Read the model definition and answer for the solid it produces. Units are mm, in the model's axes. A direction names the side the tool comes from. Give positions to 0.01 mm unless a question says otherwise; leave off trailing zeros. Order: outer loops, then holes, each group sorted by start corner. A loop starts at its lowest first (then second) coordinate and runs counter-clockwise, first axis right, second up.
Item 1: The mould has two halves that part along X. Classify faces 4 (the face through (-23.897, -34.973, 6.529)), 5 (the face through (121.398, 23, 13)), 6 (the face through (38.65, 3.02, 2.06)), 7 (the face through (-39.378, 22.614, 2.504)): +X half, -X half, draft (parallel to the pull), parting line (faces both ways), or undercut.
Item 2: Given pin 1 Ø1 at (y, z) = (-45, 17) entering from -X; pin 2 Ø1.5 at (y, z) = (-42, 13) entering from +X; pin 3 Ø1 at (x, z) = (82.5, 16.5) entering from -Y, each flat-ended and moving along its own axis, determine where each tip first touches the part or whether it passes through.
Item 3: Find the intervals of material crossed by line 1 along Y through (x, z) = (54.5, 10.75); line 2 along X through (y, z) = (-28, 18); line 3 along X through (y, z) = (-52.5, 14.5), in increasing order.
Item 4: Which of the six approach directions +Z, -Z, +X, -X, +Y, -Y give full straight-line access (tool end or side, diameter ignored) to faces 1 (the face through (96.987, -33, 13)), 2 (the face through (-35.43, -34.97, 6.61)), 3 (the face through (-38.81, 42.18, 21.93))?
Item 5: A cutting plane is placed at A-A (y = -45.5). Write down the section's boundary in (x, z), plus the area to 3 significant figures.
Item 6: A cutting plane is placed at B-B (x = 14.5). Write down the section's boundary in (y, z), plus the area to 3 significant figures.
from build123d import *

# Parameters (mm, degrees)
F0_W         = 163.3519083261
F0_H         = 45.7251667976
F1_DEPTH     = 25.4
F2_SIZE      = 5.08
F3_W         = 14.5046669376
F3_H         = 15.24
F4_DEPTH     = 70.9391236305
F5_W         = 19.3313653898
F5_H         = 15.24
F6_DEPTH     = 72.0867142081
F7_T1_DEPTH  = 39.9046669376
F7_T6_DEPTH  = 96.3391236305
F7_T12_DEPTH = 96.3391236305
F7_T18_DEPTH = 96.3391236305
F7_T24_DEPTH = 83.6391236305
F7_T29_DEPTH = 83.6391236305
F7_T34_DEPTH = 83.6391236305
F7_T39_DEPTH = 83.6391236305
F7_T44_DEPTH = 96.3391236305
F7_T50_DEPTH = 96.3391236305
F7_T56_DEPTH = 96.3391236305
F8_T1_DEPTH  = 6.4524666085
F8_T3_DEPTH  = 6.4524666085
F8_T5_DEPTH  = 85.150863787
F8_T7_DEPTH  = 45.4596645476
F8_T9_DEPTH  = 41.3682991577
F8_T14_DEPTH = 98.2150133659
F8_T19_DEPTH = 98.2150133659
F8_T24_DEPTH = 98.2150133659
F8_T29_DEPTH = 98.2150133659


# Not quite as in the source:
# - a fillet or chamfer that OpenCascade refuses, or shapes differently, is made with other operations: its cross-section is extruded or revolved along the edge and cut away or added


with BuildPart() as f1:
    # F0 (on Top) → F1 (new body)
    with BuildSketch(Plane.XY):
        with Locations((39.7221744061, 22.8625833988)):
            Rectangle(F0_W, F0_H)
    extrude(amount=F1_DEPTH)

    # F2
    f2_edges = [f1.edges().sort_by_distance(p)[0] for p in [
        (121.398129, 22.862583, 25.4),
        (121.398129, 22.862583, 0),
        (39.722174, 0, 0),
        (121.398129, 0, 12.7),
        (121.398129, 45.725167, 12.7),
        (39.722174, 45.725167, 0),
        (39.722174, 45.725167, 25.4),
        (-41.95378, 22.862583, 25.4),
        (-41.95378, 0, 12.7),
        (-41.95378, 22.862583, 0),
        (-41.95378, 45.725167, 12.7),
        (39.722174, 0, 25.4),
    ]]
    chamfer(f2_edges, length=F2_SIZE)

    # F3 (on face) → F4 (join)
    with BuildSketch(Plane.XZ):
        with Locations((-29.6214462882, 12.7)):
            Rectangle(F3_W, F3_H)
    extrude(amount=F4_DEPTH)

    # F5 (on face) → F6 (join)
    with BuildSketch(Plane.XZ):
        with Locations((106.6524458742, 12.7)):
            Rectangle(F5_W, F5_H)
    extrude(amount=F6_DEPTH)

    # F7: fillet of radius 5.08 on 5 edges, made by hand

    # F7_s2 → F7_t1 (cut)
    with BuildSketch(Plane.YZ.offset(-49.573779757)):
        with BuildLine():
            ThreePointArc((-65.8591236305, 20.32), (-69.451226079, 18.8321024484), (-70.9391236305, 15.24))
            Line((-70.9391236305, 15.24), (-70.9391236305, 20.32))
            Line((-70.9391236305, 20.32), (-65.8591236305, 20.32))
        make_face()
    extrude(amount=F7_T1_DEPTH, mode=Mode.SUBTRACT)


with BuildPart() as f7_tool4:
    # F7_s5 → F7_t6 (new body)
    with BuildSketch(Plane.XZ.offset(-12.7)):
        with BuildLine():
            ThreePointArc((-36.873779757, 15.24), (-35.3858822055, 18.8321024484), (-31.793779757, 20.32))
            Line((-31.793779757, 20.32), (-36.873779757, 20.32))
            Line((-36.873779757, 20.32), (-36.873779757, 15.24))
        make_face()
    extrude(amount=F7_T6_DEPTH)

    split(bisect_by=Plane(origin=(-18.4368898785, -18.4368898785, 0), x_dir=(0, 0, 1), z_dir=(0.7071067812, 0.7071067812, 0)), keep=Keep.TOP)

    split(bisect_by=Plane(origin=(0, -10.16, 10.16), x_dir=(1, 0, 0), z_dir=(0, -0.7071067812, 0.7071067812)), keep=Keep.TOP)


with BuildPart() as f1_1:
    add(f1.part)

    # F7_t3: cut F7_tool4
    add(f7_tool4.part, mode=Mode.SUBTRACT)


with BuildPart() as f7_tool10:
    # F7_s11 → F7_t12 (new body)
    with BuildSketch(Plane.XZ.offset(-12.7)):
        with BuildLine():
            ThreePointArc((-36.873779757, 15.24), (-35.3858822055, 18.8321024484), (-31.793779757, 20.32))
            Line((-31.793779757, 20.32), (-36.873779757, 20.32))
            Line((-36.873779757, 20.32), (-36.873779757, 15.24))
        make_face()
    extrude(amount=F7_T12_DEPTH)

    split(bisect_by=Plane(origin=(-18.4368898785, -18.4368898785, 0), x_dir=(0, 0, 1), z_dir=(-0.7071067812, -0.7071067812, 0)), keep=Keep.TOP)

    split(bisect_by=Plane(origin=(0, -10.16, 10.16), x_dir=(1, 0, 0), z_dir=(0, 0.7071067812, -0.7071067812)), keep=Keep.TOP)


with BuildPart() as f1_2:
    add(f1_1.part)

    # F7_t9: cut F7_tool10
    add(f7_tool10.part, mode=Mode.SUBTRACT)


with BuildPart() as f7_tool16:
    # F7_s17 → F7_t18 (new body)
    with BuildSketch(Plane.XZ.offset(-12.7)):
        with BuildLine():
            ThreePointArc((-36.873779757, 15.24), (-35.3858822055, 18.8321024484), (-31.793779757, 20.32))
            Line((-31.793779757, 20.32), (-36.873779757, 20.32))
            Line((-36.873779757, 20.32), (-36.873779757, 15.24))
        make_face()
    extrude(amount=F7_T18_DEPTH)

    split(bisect_by=Plane(origin=(-18.4368898785, -18.4368898785, 0), x_dir=(0, 0, 1), z_dir=(-0.7071067812, -0.7071067812, 0)), keep=Keep.TOP)

    split(bisect_by=Plane(origin=(0, -10.16, 10.16), x_dir=(1, 0, 0), z_dir=(0, -0.7071067812, 0.7071067812)), keep=Keep.TOP)


with BuildPart() as f1_3:
    add(f1_2.part)

    # F7_t15: cut F7_tool16
    add(f7_tool16.part, mode=Mode.SUBTRACT)


with BuildPart() as f7_tool22:
    # F7_s23 → F7_t24 (new body)
    with BuildSketch(Plane.XZ):
        with BuildLine():
            ThreePointArc((-27.4491128194, 5.08), (-23.857010371, 6.5678975516), (-22.3691128194, 10.16))
            Line((-22.3691128194, 10.16), (-22.3691128194, 5.08))
            Line((-22.3691128194, 5.08), (-27.4491128194, 5.08))
        make_face()
    extrude(amount=F7_T24_DEPTH)

    split(bisect_by=Plane(origin=(0, 2.54, 2.54), x_dir=(1, 0, 0), z_dir=(0, 0.7071067812, 0.7071067812)), keep=Keep.TOP)


with BuildPart() as f1_4:
    add(f1_3.part)

    # F7_t21: cut F7_tool22
    add(f7_tool22.part, mode=Mode.SUBTRACT)


with BuildPart() as f7_tool27:
    # F7_s28 → F7_t29 (new body)
    with BuildSketch(Plane.XZ):
        with BuildLine():
            ThreePointArc((-27.4491128194, 5.08), (-23.857010371, 6.5678975516), (-22.3691128194, 10.16))
            Line((-22.3691128194, 10.16), (-22.3691128194, 5.08))
            Line((-22.3691128194, 5.08), (-27.4491128194, 5.08))
        make_face()
    extrude(amount=F7_T29_DEPTH)

    split(bisect_by=Plane(origin=(0, 2.54, 2.54), x_dir=(1, 0, 0), z_dir=(0, -0.7071067812, -0.7071067812)), keep=Keep.TOP)


with BuildPart() as f1_5:
    add(f1_4.part)

    # F7_t26: cut F7_tool27
    add(f7_tool27.part, mode=Mode.SUBTRACT)


with BuildPart() as f7_tool32:
    # F7_s33 → F7_t34 (new body)
    with BuildSketch(Plane.XZ):
        with BuildLine():
            ThreePointArc((-27.4491128194, 20.32), (-23.857010371, 18.8321024484), (-22.3691128194, 15.24))
            Line((-22.3691128194, 15.24), (-22.3691128194, 20.32))
            Line((-22.3691128194, 20.32), (-27.4491128194, 20.32))
        make_face()
    extrude(amount=F7_T34_DEPTH)

    split(bisect_by=Plane(origin=(0, -10.16, 10.16), x_dir=(1, 0, 0), z_dir=(0, 0.7071067812, -0.7071067812)), keep=Keep.TOP)


with BuildPart() as f1_6:
    add(f1_5.part)

    # F7_t31: cut F7_tool32
    add(f7_tool32.part, mode=Mode.SUBTRACT)


with BuildPart() as f7_tool37:
    # F7_s38 → F7_t39 (new body)
    with BuildSketch(Plane.XZ):
        with BuildLine():
            ThreePointArc((-27.4491128194, 20.32), (-23.857010371, 18.8321024484), (-22.3691128194, 15.24))
            Line((-22.3691128194, 15.24), (-22.3691128194, 20.32))
            Line((-22.3691128194, 20.32), (-27.4491128194, 20.32))
        make_face()
    extrude(amount=F7_T39_DEPTH)

    split(bisect_by=Plane(origin=(0, -10.16, 10.16), x_dir=(1, 0, 0), z_dir=(0, -0.7071067812, 0.7071067812)), keep=Keep.TOP)


with BuildPart() as f1_7:
    add(f1_6.part)

    # F7_t36: cut F7_tool37
    add(f7_tool37.part, mode=Mode.SUBTRACT)


with BuildPart() as f7_tool42:
    # F7_s43 → F7_t44 (new body)
    with BuildSketch(Plane.XZ.offset(-12.7)):
        with BuildLine():
            ThreePointArc((-36.873779757, 10.16), (-35.3858822055, 6.5678975516), (-31.793779757, 5.08))
            Line((-31.793779757, 5.08), (-36.873779757, 5.08))
            Line((-36.873779757, 5.08), (-36.873779757, 10.16))
        make_face()
    extrude(amount=F7_T44_DEPTH)

    split(bisect_by=Plane(origin=(-18.4368898785, -18.4368898785, 0), x_dir=(0, 0, 1), z_dir=(0.7071067812, 0.7071067812, 0)), keep=Keep.TOP)

    split(bisect_by=Plane(origin=(0, 2.54, 2.54), x_dir=(1, 0, 0), z_dir=(0, -0.7071067812, -0.7071067812)), keep=Keep.TOP)


with BuildPart() as f1_8:
    add(f1_7.part)

    # F7_t41: cut F7_tool42
    add(f7_tool42.part, mode=Mode.SUBTRACT)


with BuildPart() as f7_tool48:
    # F7_s49 → F7_t50 (new body)
    with BuildSketch(Plane.XZ.offset(-12.7)):
        with BuildLine():
            ThreePointArc((-36.873779757, 10.16), (-35.3858822055, 6.5678975516), (-31.793779757, 5.08))
            Line((-31.793779757, 5.08), (-36.873779757, 5.08))
            Line((-36.873779757, 5.08), (-36.873779757, 10.16))
        make_face()
    extrude(amount=F7_T50_DEPTH)

    split(bisect_by=Plane(origin=(-18.4368898785, -18.4368898785, 0), x_dir=(0, 0, 1), z_dir=(-0.7071067812, -0.7071067812, 0)), keep=Keep.TOP)

    split(bisect_by=Plane(origin=(0, 2.54, 2.54), x_dir=(1, 0, 0), z_dir=(0, 0.7071067812, 0.7071067812)), keep=Keep.TOP)


with BuildPart() as f1_9:
    add(f1_8.part)

    # F7_t47: cut F7_tool48
    add(f7_tool48.part, mode=Mode.SUBTRACT)


with BuildPart() as f7_tool54:
    # F7_s55 → F7_t56 (new body)
    with BuildSketch(Plane.XZ.offset(-12.7)):
        with BuildLine():
            ThreePointArc((-36.873779757, 10.16), (-35.3858822055, 6.5678975516), (-31.793779757, 5.08))
            Line((-31.793779757, 5.08), (-36.873779757, 5.08))
            Line((-36.873779757, 5.08), (-36.873779757, 10.16))
        make_face()
    extrude(amount=F7_T56_DEPTH)

    split(bisect_by=Plane(origin=(-18.4368898785, -18.4368898785, 0), x_dir=(0, 0, 1), z_dir=(-0.7071067812, -0.7071067812, 0)), keep=Keep.TOP)

    split(bisect_by=Plane(origin=(0, 2.54, 2.54), x_dir=(1, 0, 0), z_dir=(0, -0.7071067812, -0.7071067812)), keep=Keep.TOP)


with BuildPart() as f1_10:
    add(f1_9.part)

    # F7_t53: cut F7_tool54
    add(f7_tool54.part, mode=Mode.SUBTRACT)

    # F8: chamfer of 5.08 on 7 edges, made by hand

    # F8_s2 → F8_t1 (cut)
    with BuildSketch(Plane(origin=(4.9133496571, 4.9133496571, -4.9133496571), x_dir=(0.7071067812, -0.7071067812, 0), z_dir=(-0.5773502692, -0.5773502692, 0.5773502692))):
        Polygon((119.5530023794, 30.9044155805), (123.1451048279, 24.6827116338), (115.960899931, 24.6827116338), align=None)
    extrude(amount=F8_T1_DEPTH, mode=Mode.SUBTRACT)

    # F8_s4 → F8_t3 (cut)
    with BuildSketch(Plane(origin=(13.3800163237, 13.3800163237, 13.3800163237), x_dir=(0.7071067812, -0.7071067812, 0), z_dir=(-0.5773502692, -0.5773502692, -0.5773502692))):
        Polygon((119.5530023794, -10.1654024249), (123.1451048279, -3.9436984783), (115.960899931, -3.9436984783), align=None)
    extrude(amount=F8_T3_DEPTH, mode=Mode.SUBTRACT)

    # F8_s6 → F8_t5 (cut)
    with BuildSketch(Plane.XZ):
        Polygon((96.9867631793, 15.24), (102.0667631793, 20.32), (96.9867631793, 20.32), align=None)
        Polygon((96.9867631793, 10.16), (102.0667631793, 5.08), (96.9867631793, 5.08), align=None)
    extrude(amount=F8_T5_DEPTH, mode=Mode.SUBTRACT)

    # F8_s8 → F8_t7 (cut)
    with BuildSketch(Plane.YZ.offset(83.9226136004)):
        Polygon((-72.0867142081, 15.24), (-67.0067142081, 20.32), (-72.0867142081, 20.32), align=None)
        Polygon((-72.0867142081, 10.16), (-67.0067142081, 5.08), (-72.0867142081, 5.08), align=None)
    extrude(amount=F8_T7_DEPTH, mode=Mode.SUBTRACT)

    # F8_s10 → F8_t9 (cut)
    with BuildSketch(Plane.XY.offset(-7.9841495789)):
        Polygon((102.0667631793, -72.0867142081), (96.9867631793, -67.0067142081), (96.9867631793, -72.0867142081), align=None)
    extrude(amount=F8_T9_DEPTH, mode=Mode.SUBTRACT)


with BuildPart() as f8_tool12:
    # F8_s13 → F8_t14 (new body)
    with BuildSketch(Plane.XZ.offset(-13.0641495789)):
        Polygon((116.3181285691, 15.24), (111.2381285691, 20.32), (116.3181285691, 20.32), align=None)
    extrude(amount=F8_T14_DEPTH)

    split(bisect_by=Plane(origin=(0, -10.16, 10.16), x_dir=(1, 0, 0), z_dir=(0, -0.7071067812, 0.7071067812)), keep=Keep.TOP)


with BuildPart() as f1_11:
    add(f1_10.part)

    # F8_t11: cut F8_tool12
    add(f8_tool12.part, mode=Mode.SUBTRACT)


with BuildPart() as f8_tool17:
    # F8_s18 → F8_t19 (new body)
    with BuildSketch(Plane.XZ.offset(-13.0641495789)):
        Polygon((116.3181285691, 15.24), (111.2381285691, 20.32), (116.3181285691, 20.32), align=None)
    extrude(amount=F8_T19_DEPTH)

    split(bisect_by=Plane(origin=(58.1590642846, -58.1590642846, 0), x_dir=(0, 0, 1), z_dir=(0.7071067812, -0.7071067812, 0)), keep=Keep.TOP)


with BuildPart() as f1_12:
    add(f1_11.part)

    # F8_t16: cut F8_tool17
    add(f8_tool17.part, mode=Mode.SUBTRACT)


with BuildPart() as f8_tool22:
    # F8_s23 → F8_t24 (new body)
    with BuildSketch(Plane.XZ.offset(-13.0641495789)):
        Polygon((116.3181285691, 10.16), (111.2381285691, 5.08), (116.3181285691, 5.08), align=None)
    extrude(amount=F8_T24_DEPTH)

    split(bisect_by=Plane(origin=(0, 2.54, 2.54), x_dir=(1, 0, 0), z_dir=(0, -0.7071067812, -0.7071067812)), keep=Keep.TOP)


with BuildPart() as f1_13:
    add(f1_12.part)

    # F8_t21: cut F8_tool22
    add(f8_tool22.part, mode=Mode.SUBTRACT)


with BuildPart() as f8_tool27:
    # F8_s28 → F8_t29 (new body)
    with BuildSketch(Plane.XZ.offset(-13.0641495789)):
        Polygon((116.3181285691, 10.16), (111.2381285691, 5.08), (116.3181285691, 5.08), align=None)
    extrude(amount=F8_T29_DEPTH)

    split(bisect_by=Plane(origin=(58.1590642846, -58.1590642846, 0), x_dir=(0, 0, 1), z_dir=(0.7071067812, -0.7071067812, 0)), keep=Keep.TOP)


with BuildPart() as f1_14:
    add(f1_13.part)

    # F8_t26: cut F8_tool27
    add(f8_tool27.part, mode=Mode.SUBTRACT)


solid = f1_14.part
Response values:
1. face 4: undercut
1. face 5: +X half
1. face 6: draft
1. face 7: -X half
2. pin 1: stops at x = -36.72
2. pin 2: stops at x = 116.32
2. pin 3: stops at y = 0
3. line 1: y = 0 to 45.73
3. line 2: x = -36.06 to -23.18, 99.75 to 113.56
3. line 3: x = -36.87 to -22.37, 96.99 to 116.32
4. face 1: +Z, -Z, -Y
4. face 2: -Z, -X, -Y
4. face 3: +Z, -X, +Y
5. outline: (-36.87, 10.16) arc R5.08 ccw to (-31.79, 5.08) - (-27.45, 5.08) arc R5.08 ccw to (-22.37, 10.16) - (-22.37, 15.24) arc R5.08 ccw to (-27.45, 20.32) - (-31.79, 20.32) arc R5.08 ccw to (-36.87, 15.24) - close; (96.99, 10.16) - (102.07, 5.08) - (111.24, 5.08) - (116.32, 10.16) - (116.32, 15.24) - (111.24, 20.32) - (102.07, 20.32) - (96.99, 15.24) - close
5. area: 442 mm2
6. outline: (0, 5.08) - (5.08, 0) - (40.65, 0) - (45.73, 5.08) - (45.73, 20.32) - (40.65, 25.4) - (5.08, 25.4) - (0, 20.32) - close
6. area: 1,110 mm2
